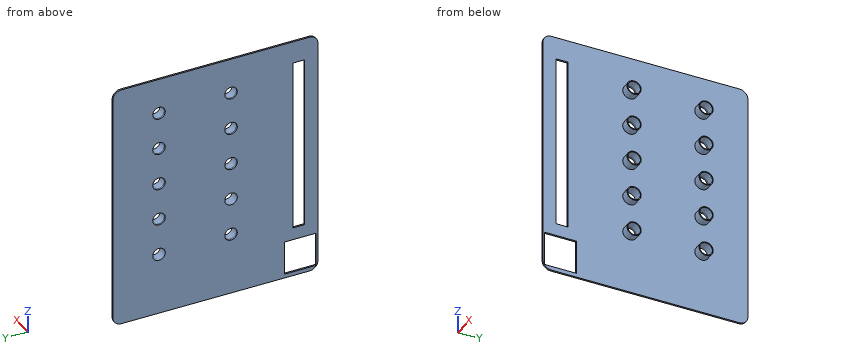
Autodesk Inventor part; units mm, degrees
ref_plane "YZ Plane" through (0, 0, 0) normal (1, 0, 0) x (0, 1, 0)
ref_plane "XZ Plane" through (0, 0, 0) normal (0, 1, 0) x (-1, 0, 0)
ref_plane "XY Plane" through (0, 0, 0) normal (0, 0, 1) x (1, 0, 0)
sketch "Sketch1" plane through (0, 0, 0) normal (1, 0, 0) x (0, 1, 0)
  line L0 (0, 0) -> (245, 0)
  line L1 (245, 0) -> (245, -298.222)
  line L2 (245, -298.222) -> (0, -298.222)
  line L3 (0, -298.222) -> (0, 0)
  dimension "d0" = 245
  dimension "d1" = 298.222
extrude "Extrusion1" add sketch "Sketch1" along normal blind 2
sketch "Sketch2" plane through (2, 0, 0) normal (1, 0, 0) x (0, 0, -1)
  line L0 (252.355, 2) -> (293.422, 2)
  line L1 (293.422, 2) -> (293.422, 40)
  line L2 (293.422, 40) -> (252.355, 40)
  line L3 (252.355, 40) -> (252.355, 2)
  line L4 (0, 0) -> (298.222, 0)
  line L5 (0, 245) -> (0, 0)
  line L6 (298.222, 0) -> (298.222, 245)
  dimension "d4" = 2
  dimension "d6" = 38
  dimension "d7" = 41.067
  dimension "d8" = 4.8
extrude "Extrusion2" cut sketch "Sketch2" against normal blind 10
sketch "Sketch3" plane through (2, 0, 0) normal (1, 0, 0) x (0, 0, -1)
  line L0 (237.355, 29.8) -> (27, 29.8)
  line L1 (27, 29.8) -> (27, 15.8)
  line L2 (27, 15.8) -> (237.355, 15.8)
  line L3 (237.355, 15.8) -> (237.355, 29.8)
  line L4 (252.355, 2) -> (252.355, 40)
  line L5 (0, 0) -> (298.222, 0)
  line L6 (0, 245) -> (0, 0)
  dimension "d11" = 15
  dimension "d12" = 15.8
  dimension "d13" = 14
  dimension "d14" = 27
extrude "Extrusion3" cut sketch "Sketch3" against normal blind 10
sketch "Sketch4" plane through (0, 0, 0) normal (-1, 0, 0) x (0, 0, 1)
  circle A0 centre (-223.222, 190) radius 7.5
  line L0 (0, 245) -> (-298.222, 245)
  line L1 (-298.222, 245) -> (-298.222, 0)
  point P0 (0, 0)
  dimension "d17" = 15
  dimension "d18" = 55
  dimension "d19" = 75
extrude "Extrusion4" cut sketch "Sketch4" against normal blind 10
pattern_linear "Rectangular Pattern1" count 5 spacing 45 along (0, 0, 1) of "Extrusion4"
pattern_linear "Rectangular Pattern2" count 2 spacing 86.16 along (0, -1, 0) of "Extrusion4", "Rectangular Pattern1"
sketch "Sketch5" plane through (2, 0, 0) normal (1, 0, 0) x (0, 0, -1)
  circle A0 centre (43.222, 190) radius 7.5
  circle A1 centre (43.222, 190) radius 7.5
  circle A2 centre (43.222, 190) radius 8.5
  point P0 (0, 0)
  dimension "d28" = 17
extrude "Extrusion5" add sketch "Sketch5" along normal blind 10
pattern_linear "Rectangular Pattern3" count 5 spacing 45 along (0, 0, -1) of "Extrusion5"
pattern_linear "Rectangular Pattern4" count 2 spacing 86.16 along (0, -1, 0) of "Extrusion5", "Rectangular Pattern3"
fillet "Fillet1" radius 10 4 edges at (1, 245, 0) (1, 245, -298.222) (1, 0, -298.222) (1, 0, 0)
properties part number "frount glass" material "Glass"
Verification items for the finished model (mm, model axes). Coordinates: 2 decimals unless noted, no trailing zeros. Write each loop counter-clockwise with the first axis right and the second up, starting at its lowest first coordinate (ties: lowest second). Pieces come first, ordered by that corner, then holes. Notation, with made-up numbers: M 50.5,-4 L 82.5,-4 A19 cw 82.5,4 Z; hole C 85.25,37.5 d10. An arc over 180 degrees is marked long. Use a Markdown table: item, result.
Q1. Sectioned sample at A-A, the plane x = 4.5. Count the separate pieces of the cut face and the enclosed holes in it, plus the area to 3 significant figures.
Reply:
| item | result |
|---|---|
| separate pieces | 10 |
| enclosed holes | 10 |
| area | 503 mm² |
Q2. Go/stop test with flat-tipped pins: P1, Ø12, axis at y = 103.84, z = -133.222, coming from the +X side; P2, Ø12, axis at y = 130, z = -257, coming from the +X side. Record where each tip stops, or that it passes through.
Reply:
| item | result |
|---|---|
| P1 | passes through |
| P2 | stops at x = 2 |
Q3. Sectioned sample at C-C, the plane y = 210. Record the boundary of the cut face in (x, z), plus the area to 3 significant figures.
Reply:
| item | result |
|---|---|
| outline | M 0,-298.22 L 2,-298.22 L 2,0 L 0,0 Z |
| area | 596 mm² |
Q4. Thickness scan on line 1 (Z direction, x = 1.55, y = 103.84); line 2 (Y direction, x = 5.75, z = -86); line 3 (Y direction, x = 6, z = -177). Record the ranges inside material, lowest first.
Reply:
| item | result |
|---|---|
| line 1 | z = -298.22 to -230.72, -215.72 to -185.72, -170.72 to -140.72, -125.72 to -95.72, -80.72 to -50.72, -35.72 to 0 |
| line 2 | y = 95.64 to 96.68, 111 to 112.04, 181.8 to 182.84, 197.16 to 198.2 |
| line 3 | y = 95.43 to 96.44, 111.24 to 112.25, 181.59 to 182.6, 197.4 to 198.41 |
